Here's how the part is built. I have some questions about the finished solid (model axes, mm). Round coordinates to 2 decimals unless told otherwise and drop trailing zeros. Loops run counter-clockwise (first coordinate to the right, second up) from the corner with the lowest first, then second, coordinate; pieces in that order, holes last. Notation, with made-up numbers: (89.5, 73.25) -> (138.5, 73.25) arc R35 cw to (138.5, 110.25) -> close; hole circle Ø4 at (34.25, -10.75). An arc over 180 degrees is marked (long way). Use one line per item in the form item = value. Start each with the question number.
Item 1: If we section it at A-A (z = -23): Write out the boundary of the cut face in (x, y).
Item 2: If we section it at B-B (z = 131): Write out the boundary of the cut face in (x, y).
Item 3: I'm going to push flat-ended pins straight in: pin 1 Ø9 at (x, y) = (1, -2.5) entering from -Z; pin 2 Ø4 at (y, z) = (0, 134.5) entering from -X; pin 3 Ø0.6 at (x, y) = (6.5, 2) entering from -Z; pin 4 Ø5.5 at (y, z) = (0.5, -20) entering from -X. Where does each tip first touch, or does it pass through?
Item 4: If I drill on L1, parallel to Z at x = 5.4, y = 0; L2, parallel to Z at x = 1, y = 0; L3, parallel to Z at x = -4.4, y = 0, over which ranges is the centre line in solid material (lowest first)? Write a range as [from, to].
Autodesk Inventor part; units mm, degrees
ref_plane "YZ Plane" through (0, 0, 0) normal (1, 0, 0) x (0, 1, 0)
ref_plane "XZ Plane" through (0, 0, 0) normal (0, 1, 0) x (-1, 0, 0)
ref_plane "XY Plane" through (0, 0, 0) normal (0, 0, 1) x (1, 0, 0)
sketch "Esboço1" plane through (0, 0, 0) normal (0, 0, 1) x (1, 0, 0)
  circle A0 centre (0, 0) radius 8.5
  dimension "d0" = 17
extrude "Extrusão1" add sketch "Esboço1" against normal blind 10
sketch "Esboço2" plane through (0, 0, 0) normal (0, 0, 1) x (1, 0, 0)
  circle A0 centre (0, 0) radius 8.5
  circle A1 centre (0, 0) radius 5
  dimension "d3" = 10
extrude "Extrusão2" add sketch "Esboço2" along normal blind 325 contours A1
sketch "Esboço3" plane through (0, 0, -10) normal (0, 0, -1) x (-1, 0, 0)
  circle A0 centre (0, 0) radius 8.5
  circle A1 centre (0, 0) radius 8
  dimension "d6" = 16
extrude "Extrusão3" add sketch "Esboço3" along normal blind 18 contours A1
sketch "Esboço4" plane through (0, 0, -28) normal (0, 0, -1) x (-1, 0, 0)
  circle A0 centre (0, 0) radius 8
  circle A1 centre (0, 0) radius 8
  line L0 (-4, 6.9282) -> (-4, -6.9282)
  line L1 (4, 6.9282) -> (4, -6.9282)
  arc A2 (-4, -6.9282) -> (4, -6.9282) centre (0, 0) ccw
  arc A3 (4, 6.9282) -> (-4, 6.9282) centre (0, 0) ccw
  point P0 (-4, -6.9282)
  dimension "d9" = 4
  dimension "d10" = 4
extrude "Extrusão4" cut sketch "Esboço4" against normal blind 15 contours L1 A0 L0
sketch "Esboço6" plane through (0, 0, -28) normal (0, 0, -1) x (-1, 0, 0)
  line L0 (-4, -6.9282) -> (-4, 6.9282)
  arc A0 (-4, 6.9282) -> (-4, -6.9282) centre (0, 0) ccw
  circle A1 centre (0, 0) radius 8
  line L1 (-6, 5.2915) -> (-6, -5.2915)
  line L2 (6, 5.2915) -> (6, -5.2915)
  arc A2 (-6, 5.2915) -> (-6, -5.2915) centre (0, 0) ccw
  arc A3 (6, -5.2915) -> (6, 5.2915) centre (0, 0) ccw
  point P0 (6, -5.2915)
  dimension "d15" = 6
  dimension "d16" = 6
extrude "Extrusão5" cut sketch "Esboço6" against normal blind 12 contours A0 L1 | L2 A1
sketch "Esboço7" plane through (0, 0, 0) normal (1, 0, 0) x (0, 1, 0)
  circle A0 centre (0, -23) radius 3
  line L0 (-6.9282, -28) -> (6.9282, -28)
  point P0 (0, 0)
  dimension "d19" = 5
  dimension "d20" = 6
extrude "Extrusão6" cut sketch "Esboço7" along normal through all both and the other way through all
chamfer "Chanfro1" distance 0.5 angle 45 4 edges at (-5.0665, -6.1911, -28) (-5.0665, 6.1911, -28) (5.0665, -6.1911, -28) (5.0665, 6.1911, -28)
fillet "Arredondamento1" radius 4 1 edges at (-5, 0, 325)
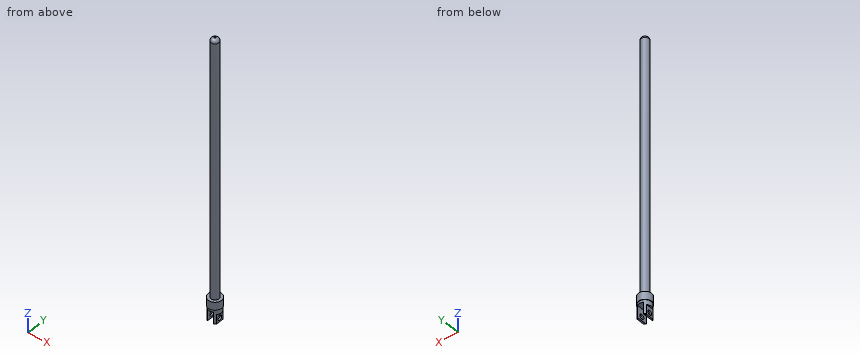
Values found:
q1.outline = (-6, -5.29) arc R8 ccw to (-4, -6.93) -> (-4, -3) -> (-6, -3) -> close; (-6, 3) -> (-4, 3) -> (-4, 6.93) arc R8 ccw to (-6, 5.29) -> close; (4, -6.93) arc R8 ccw to (6, -5.29) -> (6, -3) -> (4, -3) -> close; (4, 3) -> (6, 3) -> (6, 5.29) arc R8 ccw to (4, 6.93) -> close
q2.outline = circle Ø10 at (0, 0)
q3.pin_1 = -28
q3.pin_2 = -5
q3.pin_3 = -16
q3.pin_4 = -6
q4.L1 = [-28, -26], [-20, 0]
q4.L2 = [-13, 325]
q4.L3 = [-28, -26], [-20, 323.11]
